Print and shaded views of the part. All mm, measured from the part's lowest x, y and z. Coordinates: 2 decimals unless noted, no trailing zeros. Order: outer loops, then holes, each group sorted by start corner. A loop starts at its lowest first (then second) coordinate and runs counter-clockwise, first axis right, second up. Notation, with made-up numbers: M 9,-36.5 L 35,-36.5 A18 cw 35,-9.5 Z; hole C 23,-13.75 d5. An arc over 180 degrees is marked long. One line per item, written item: value.
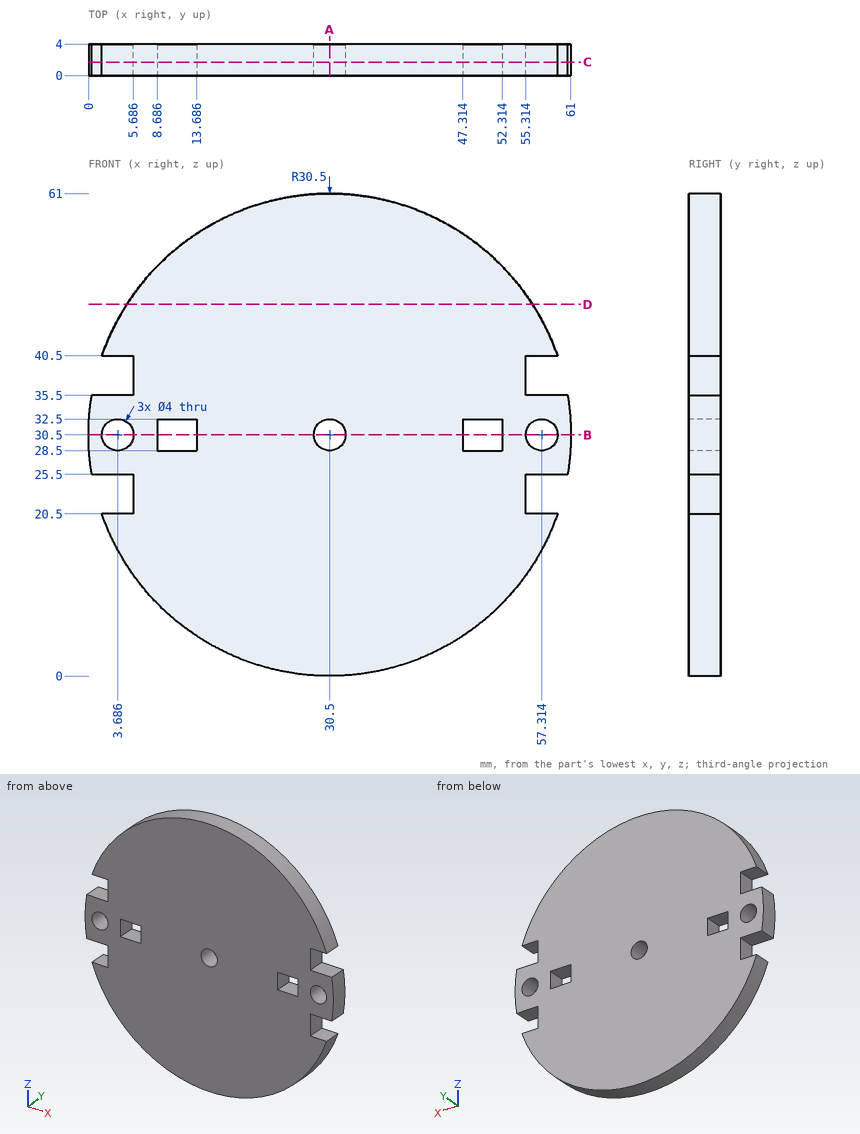
Q1. Slice it at C-C (y = 1.7). List the corners of the cut face in (x, z).
Recorded:
outline: M 0.41,25.5 L 5.69,25.5 L 5.69,20.5 L 1.69,20.5 A30.5 ccw 59.31,20.5 L 55.31,20.5 L 55.31,25.5 L 60.59,25.5 A30.5 ccw 60.59,35.5 L 55.31,35.5 L 55.31,40.5 L 59.31,40.5 A30.5 ccw 1.69,40.5 L 5.69,40.5 L 5.69,35.5 L 0.41,35.5 A30.5 ccw Z; hole C 3.69,30.5 d4; hole M 8.69,28.5 L 13.69,28.5 L 13.69,32.5 L 8.69,32.5 Z; hole C 30.5,30.5 d4; hole M 47.31,28.5 L 52.31,28.5 L 52.31,32.5 L 47.31,32.5 Z; hole C 57.31,30.5 d4
Q2. Slice it at D-D (z = 47). List the corners of the cut face in (x, y), plus the area to 3 significant figures.
Recorded:
outline: M 4.85,0 L 56.15,0 L 56.15,4 L 4.85,4 Z
area: 205 mm^2
Q3. Slice it at B-B (z = 30.5). List the corners of the cut face in (x, y).
Recorded:
outline: M 0,0 L 1.69,0 L 1.69,4 L 0,4 Z; M 5.69,0 L 8.69,0 L 8.69,4 L 5.69,4 Z; M 13.69,0 L 28.5,0 L 28.5,4 L 13.69,4 Z; M 32.5,0 L 47.31,0 L 47.31,4 L 32.5,4 Z; M 52.31,0 L 55.31,0 L 55.31,4 L 52.31,4 Z; M 59.31,0 L 61,0 L 61,4 L 59.31,4 Z
Q4. Slice it at A-A (x = 30.5). List the corners of the cut face in (y, z).
Recorded:
outline: M 0,0 L 4,0 L 4,28.5 L 0,28.5 Z; M 0,32.5 L 4,32.5 L 4,61 L 0,61 Z
Q5. Drill centre lines: line 1 along X through (y, z) = (1.8, 30.5); line 2 along Z through (x, y) = (5, 2.1); line 3 along Z through (x, y) = (35.5, 2.05). Where is each one in solid material? Low to high.
Recorded:
line 1: x = 0 to 1.69, 5.69 to 8.69, 13.69 to 28.5, 32.5 to 47.31, 52.31 to 55.31, 59.31 to 61
line 2: z = 13.77 to 20.5, 25.5 to 28.99, 32.01 to 35.5, 40.5 to 47.23
line 3: z = 0.41 to 60.59
Q6. Pin check, flat tips, straight feed: pin 1 Ø2 at (x, y) = (3.5, 2.5) entering from -Z (1 decimal); pin 2 Ø2 at (y, z) = (1.5, 31) entering from -X; pin 3 Ø1.2 at (x, y) = (12, 2.5) entering from +Z (3 decimals). Stop position of each tip, or through.
Recorded:
pin 1: stops at z = 14.6
pin 2: stops at x = 0
pin 3: stops at z = 55.195
